Could you check a few things on this model? Use its own coordinates, in mm. Face numbers are marked on the shaded views. A direction names the side the tool comes from. Round coordinates to 2 decimals unless told otherwise and drop trailing zeros. Write each loop counter-clockwise with the first axis right and the second up, starting at its lowest first coordinate (ties: lowest second). Pieces come first, ordered by that corner, then holes. Notation, with made-up numbers: (78.5, 12.5) -> (88.5, 12.5) arc R12 cw to (88.5, 23.5) -> close; hole circle Ø9 at (40, 59.25). An arc over 180 degrees is marked (long way). Return JSON: item names as keys, results as strings.
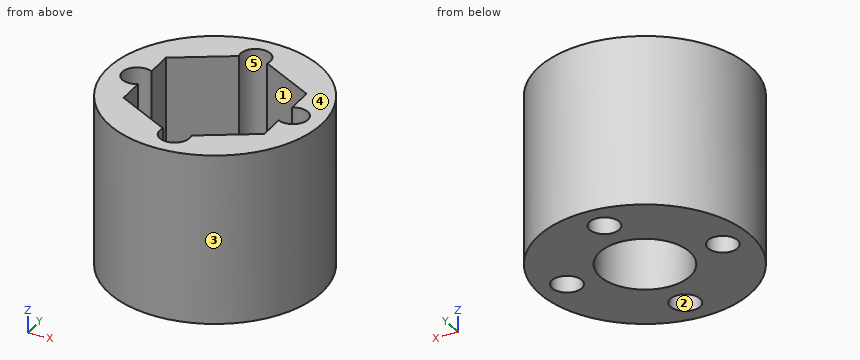
from build123d import *

# Parameters (mm, degrees)
SKETCH1_R           = 10
SKETCH1_R_2         = 1.4
SKETCH1_R_3         = 4.25
BOSS_EXTRUDE1_DEPTH = 16
CUT_EXTRUDE1_DEPTH  = 8.5


with BuildPart() as part:
    # Sketch1 → Boss-Extrude1 (new body)
    with BuildSketch(Plane.XY):
        Circle(SKETCH1_R)
        with Locations((0, 7.25)):
            Circle(SKETCH1_R_2, mode=Mode.SUBTRACT)
        Circle(SKETCH1_R_3, mode=Mode.SUBTRACT)
        with Locations((7.25, 0)):
            Circle(SKETCH1_R_2, mode=Mode.SUBTRACT)
        with Locations((0, -7.25)):
            Circle(SKETCH1_R_2, mode=Mode.SUBTRACT)
        with Locations((-7.25, 0)):
            Circle(SKETCH1_R_2, mode=Mode.SUBTRACT)
    extrude(amount=BOSS_EXTRUDE1_DEPTH)

    # Sketch2 → Cut-Extrude1 (cut)
    with BuildSketch(Plane.XY.offset(16)):
        Polygon((0, 7.563288526), (-6.55, 3.781644263), (-6.55, -3.781644263), (0, -7.563288526), (6.55, -3.781644263), (6.55, 3.781644263), align=None)
    extrude(amount=-CUT_EXTRUDE1_DEPTH, mode=Mode.SUBTRACT)


solid = part.part
1) I want a section at A-A, the plane y = 0. Please give me the cut outline in (x, z), and give its area (3 significant figures).
Return value:
{"outline": "(-10, 0) -> (-8.65, 0) -> (-8.65, 16) -> (-10, 16) -> close; (-5.85, 0) -> (-4.25, 0) -> (-4.25, 7.5) -> (-5.85, 7.5) -> close; (4.25, 0) -> (5.85, 0) -> (5.85, 7.5) -> (4.25, 7.5) -> close; (8.65, 0) -> (10, 0) -> (10, 16) -> (8.65, 16) -> close", "area": "67.2 mm²"}
2) I want a section at D-D, the plane z = 9.75. Please give me the cut outline in (x, y).
Return value:
{"outline": "circle Ø20 at (0, 0); hole (-6.55, -3.78) -> (-1.33, -6.8) arc R1.4 ccw (long way) to (1.33, -6.8) -> (6.55, -3.78) -> (6.55, -1.21) arc R1.4 ccw (long way) to (6.55, 1.21) -> (6.55, 3.78) -> (1.33, 6.8) arc R1.4 ccw (long way) to (-1.33, 6.8) -> (-6.55, 3.78) -> (-6.55, 1.21) arc R1.4 ccw (long way) to (-6.55, -1.21) -> close"}
3) Will these pins go through, and if not, where does the flat tip stop? pin 1 Ø1 at (x, z) = (-3.5, 6) entering from +Y; pin 2 Ø6.5 at (x, y) = (1.5, -2) entering from +Z; pin 3 Ø1.3 at (y, z) = (-2.5, 12) entering from +X; pin 4 Ø3.5 at (x, y) = (7.25, 0) entering from +Z.
Return value:
{"pin 1": "y = 9.54", "pin 2": "z = 7.5", "pin 3": "x = 9.83", "pin 4": "z = 16"}
4) For the marked faces 1 and 2, which set-ups out of +Z, -Z, +X, -X, +Y, -Y let a thin tool reach every point of the face, with its end or its side?
Return value:
{"face 1": "+Z", "face 2": "+Z, -Z"}
5) Thinking about a two-plate mould opening in Y: for the marked faces 3, 4 and 5, which applies, pulls with the +Y half, pulls with the -Y half, needs draft (parallel to the pull), parting line crosses it, or undercut?
Return value:
{"face 3": "parting line crosses it", "face 4": "needs draft", "face 5": "undercut"}
6) I want a section at B-B, the plane z = 7. Please give me the cut outline in (x, y), and give its area (3 significant figures).
Return value:
{"outline": "circle Ø20 at (0, 0); hole circle Ø2.8 at (-7.25, 0); hole circle Ø8.5 at (0, 0); hole circle Ø2.8 at (0, -7.25); hole circle Ø2.8 at (0, 7.25); hole circle Ø2.8 at (7.25, 0)", "area": "233 mm²"}
7) If I drill on probe 1 along Y at (x, z) = (0, 5.5); probe 2 along Z at (x, y) = (-3.5, 5.5); probe 3 along X at (y, z) = (0.25, 6.25), over which ranges is the centre line in solid material (lowest first)? Write a range as [from, to].
Return value:
{"probe 1": "[-10, -8.65], [-5.85, -4.25], [4.25, 5.85], [8.65, 10]", "probe 2": "[0, 7.5]", "probe 3": "[-10, -8.63], [-5.87, -4.24], [4.24, 5.87], [8.63, 10]"}
